Model file for the job. Use its own axes, mm. Give positions to 0.01 mm unless a question says otherwise; leave off trailing zeros. Loops run counter-clockwise (first coordinate to the right, second up) from the corner with the lowest first, then second, coordinate; pieces in that order, holes last. Notation, with made-up numbers: (38.25, 58) - (47.25, 58) arc R19 ccw to (47.25, 92) - close; hole circle Ø8 at (49, 78.25). An arc over 180 degrees is marked (long way). Answer as CSV lines item,"result". Start each with the question number.
Item 1: Saw through at B-B on x = 190.5. Give the cut face in (y, z) (3 decimals).
Item 2: Drill centre lines: L1, parallel to X at y = 204, z = 8.65 (3 decimals); L2, parallel to Y at x = 198, z = 13.75 (3 decimals); L3, parallel to Z at x = 286, y = 16.5. Where is each one in solid material? Low to high. Write a range as from..to.
Item 3: Saw through at A-A on z = 11.5. Give the cut face in (x, y) (3 decimals).
Item 4: Saw through at C-C on y = 185.5. Give the cut face in (x, z) (3 decimals).
Item 5: Pin check, flat tips, straight feed: pin 1 (5 mm diameter, centred on y = 84, z = 13, fed in from +X); pin 2 (5 mm diameter, centred on x = 203, y = 141.5, fed in from +Z); pin 3 (5 mm diameter, centred on x = 291, y = 204, fed in from -Z); pin 4 (3 mm diameter, centred on y = 84, z = 13, fed in from -X). Stop position of each tip, or through.
Item 6: Saw through at D-D on x = 235.5. Give the cut face in (y, z).
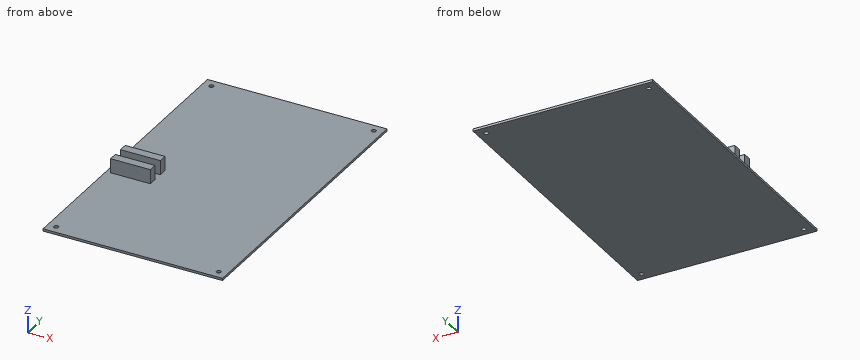
from build123d import *

# Parameters (mm, degrees)
SKETCH001_W      = 126.265
SKETCH001_H      = 210
SKETCH001_R      = 1.6
EXTRUDE001_DEPTH = 1.6
SKETCH006_W      = 28
SKETCH006_H      = 6
EXTRUDE006_DEPTH = 10


with BuildPart() as extrude001:
    # Sketch001 → Extrude001 (new body)
    with BuildSketch(Plane.XY.offset(8)):
        with Locations((233.8675, 105)):
            Rectangle(SKETCH001_W, SKETCH001_H)
        with Locations((176.735, 204)):
            Circle(SKETCH001_R, mode=Mode.SUBTRACT)
        with Locations((291, 204)):
            Circle(SKETCH001_R, mode=Mode.SUBTRACT)
        with Locations((291, 6)):
            Circle(SKETCH001_R, mode=Mode.SUBTRACT)
        with Locations((176.735, 6)):
            Circle(SKETCH001_R, mode=Mode.SUBTRACT)
    extrude(amount=EXTRUDE001_DEPTH)


with BuildPart() as ula8:
    # Sketch006 (on Face10 of Extrude001) → Extrude006 (new body)
    with BuildSketch(Plane.XY.offset(9.6)):
        with Locations((187.88, 96.255)):
            Rectangle(SKETCH006_W, SKETCH006_H)
        with Locations((187.88, 83.555)):
            Rectangle(SKETCH006_W, SKETCH006_H)
    extrude(amount=EXTRUDE006_DEPTH)

    # Fusion003: union Extrude001
    add(extrude001.part)


solid = ula8.part
Responses:
1,outline,"(0, 8) - (210, 8) - (210, 9.6) - (99.255, 9.6) - (99.255, 19.6) - (93.255, 19.6) - (93.255, 9.6) - (86.555, 9.6) - (86.555, 19.6) - (80.555, 19.6) - (80.555, 9.6) - (0, 9.6) - close"
2,L1,"170.735..175.135, 178.335..289.4, 292.6..297"
2,L2,"80.555..86.555, 93.255..99.255"
2,L3,"8..9.6"
3,outline,"(173.88, 80.555) - (201.88, 80.555) - (201.88, 86.555) - (173.88, 86.555) - close; (173.88, 93.255) - (201.88, 93.255) - (201.88, 99.255) - (173.88, 99.255) - close"
4,outline,"(170.735, 8) - (297, 8) - (297, 9.6) - (170.735, 9.6) - close"
5,pin 1,"x = 201.88"
5,pin 2,"z = 9.6"
5,pin 3,"z = 8"
5,pin 4,"x = 173.88"
6,outline,"(0, 8) - (210, 8) - (210, 9.6) - (0, 9.6) - close"
